For this review, use the dimensioned drawing (mm, ordinates from the lowest corner) and the shaded views. A direction names the side the tool comes from. Coordinates: 2 decimals unless noted, no trailing zeros. Write each loop counter-clockwise with the first axis right and the second up, starting at its lowest first coordinate (ties: lowest second). Pieces come first, ordered by that corner, then holes.
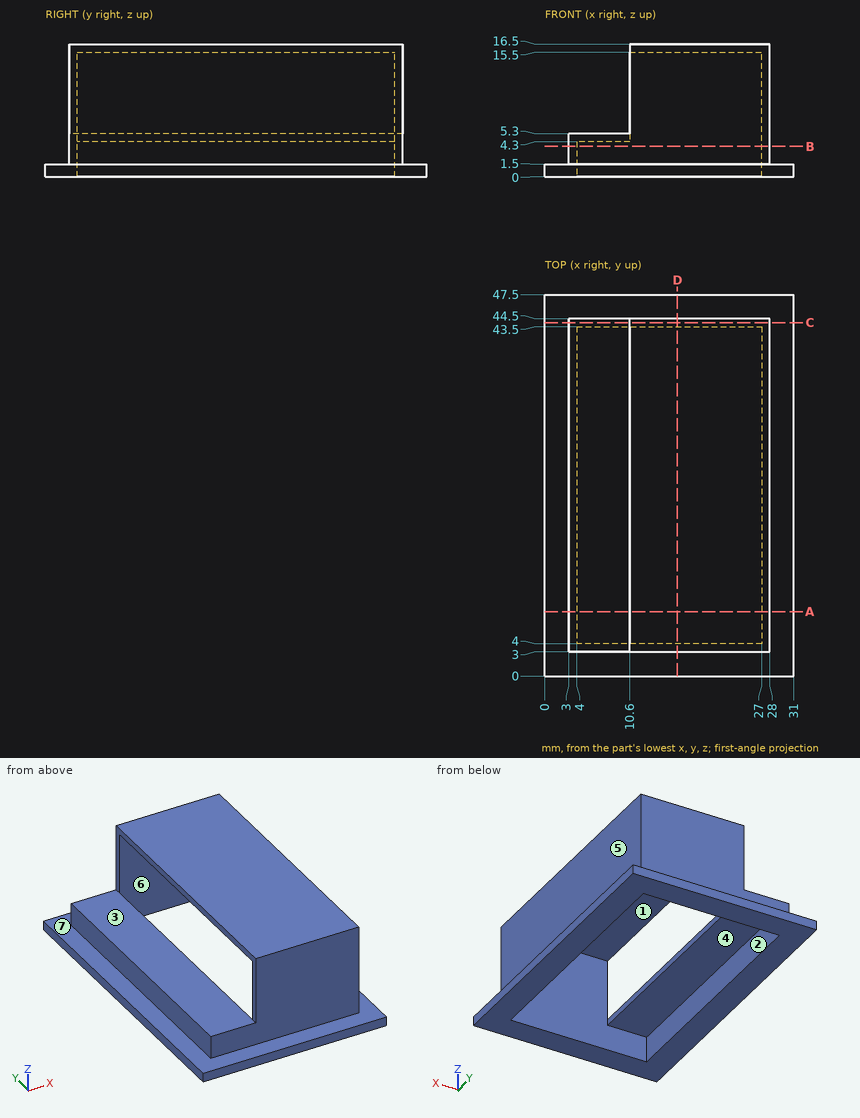
(1) Insertion check: pin 1 Ø3.5 at (y, z) = (22, 12.5) entering from -X; pin 2 Ø3 at (x, z) = (19, 4) entering from +Y; pin 3 Ø8 at (x, y) = (18.5, 24.5) entering from -Z. Each pin has a flat end and moves straight along its axis. Give the tip position at first contact, or say it passes through.
(2) Mouldability with a two-part tool opening along X and no side actions: class the marked faces 4, 5, 6 and 7 as +X half, -X half, draft (parallel to the pull), parting line (faces both ways), or undercut.
(3) Wall thickness on line 1 (Y direction, x = 22, z = 8.75); line 2 (X direction, y = 42, z = 2); line 3 (X direction, y = 29.5, z = 1): over which ranges is each line inside the solid? List them lowest first.
(4) Consider section C-C (y = 44). Give the boundary of the cut face in (x, z), plus the area to 3 significant figures.
(5) Consider section B-B (z = 3.75). Give the boundary of the cut face in (x, y).
(6) Consider section A-A (y = 8). Give the boundary of the cut face in (x, z).
(7) For the marked faces 1, 2 and 3, list the 3-axis set-ups (+Z, -Z, +X, -X, +Y, -Y) from which the entire face can be reached by the end or side of a thin tool; tool diameter is ignored.
(8) Consider section D-D (x = 16.5). Give the boundary of the cut face in (y, z).
Results:
1. pin 1: stops at x = 27
1. pin 2: stops at y = 44.5
1. pin 3: stops at z = 15.5
2. face 4: undercut
2. face 5: +X half
2. face 6: undercut
2. face 7: draft
3. line 1: y = 3 to 4, 43.5 to 44.5
3. line 2: x = 3 to 4, 27 to 28
3. line 3: x = 0 to 4, 27 to 31
4. outline: (0, 0) - (31, 0) - (31, 1.5) - (28, 1.5) - (28, 16.5) - (10.6, 16.5) - (10.6, 5.3) - (3, 5.3) - (3, 1.5) - (0, 1.5) - close
4. area: 336 mm2
5. outline: (3, 3) - (28, 3) - (28, 44.5) - (3, 44.5) - close; hole (4, 4) - (27, 4) - (27, 43.5) - (4, 43.5) - close
6. outline: (0, 0) - (4, 0) - (4, 4.3) - (10.6, 4.3) - (10.6, 5.3) - (3, 5.3) - (3, 1.5) - (0, 1.5) - close; (10.6, 15.5) - (27, 15.5) - (27, 0) - (31, 0) - (31, 1.5) - (28, 1.5) - (28, 16.5) - (10.6, 16.5) - close
7. face 1: -Z, -X
7. face 2: -Z
7. face 3: +Z, -X, +Y, -Y
8. outline: (0, 0) - (4, 0) - (4, 15.5) - (43.5, 15.5) - (43.5, 0) - (47.5, 0) - (47.5, 1.5) - (44.5, 1.5) - (44.5, 16.5) - (3, 16.5) - (3, 1.5) - (0, 1.5) - close
